Source: CAD feature listing. Evaluate the final solid. Frame: model axes, mm. A direction names the side the tool comes from. Coordinates: 2 decimals unless noted, no trailing zeros. Write each loop counter-clockwise with the first axis right and the second up, starting at its lowest first coordinate (ties: lowest second). Pieces come first, ordered by that corner, then holes. Notation, with made-up numbers: M -8.5,45 L -0.5,45 A20 cw -0.5,74 Z; hole C 47.5,0.25 d8. An arc over 180 degrees is marked long. Write item = value, one per line. Start each with the question number.
1. Section query C-C (z = 0). Output: boundary loops of the cut face in (x, y).
2. Access query for faces 3 (the face through (9.593, 4.93, 1.956)), 4 (the face through (1.26, 14.93, -0.17)). Directions: +Z, -Z, +X, -X, +Y, -Y. A direction counts if a zero-diameter tool reaches every point of the face in a straight line with its end or side. Return the directions, or none.
3. Section query D-D (z = 10). Output: boundary loops of the cut face in (x, y).
4. Line query: line 1 along X through (y, z) = (12.5, 0); line 2 along Y through (x, z) = (31, 13.5); line 3 along Z through (x, y) = (-1, 13.5). Output: solid intervals per line, ascending.
5. Section query A-A (x = 0). Output: boundary loops of the cut face in (y, z), then the cut area to 3 significant figures.
6. Pull-direction query (Z, two-part tool) for faces 1 (the face through (9.55, 4.93, -1.97)), 2 (the face through (18, 10, -18)); classes: pulls with the +Z half, pulls with the -Z half, needs draft (parallel to the pull), parting line crosses it, or undercut.
7. Pin query (flat end, axial travel): pin 1 Ø6 at (y, z) = (8, -5) entering from +X; pin 2 Ø2.5 at (y, z) = (6.5, 0) entering from +X; pin 3 Ø5 at (y, z) = (2.5, -17) entering from -X. Return the tip coordinate at first contact, or that it passes through.
```python
from build123d import *

# Parameters (mm, degrees)
SKETCH1_R           = 25
BOSS_EXTRUDE1_DEPTH = 10
SKETCH2_R           = 34
SKETCH2_R_2         = 1.27
BOSS_EXTRUDE2_DEPTH = 10
SKETCH3_R           = 3
CUT_EXTRUDE1_DEPTH  = 53.076866265


with BuildPart() as part:
    # Sketch1 → Boss-Extrude1 (new body)
    with BuildSketch(Plane(origin=(0, 0, 0), x_dir=(1, 0, 0), z_dir=(0, 1, 0))):
        with Locations(Location((0, 0, 0), (0, 0, 270))):
            Circle(SKETCH1_R)
        with BuildLine():
            Line((-1.5, 11), (1.5, 11))
            Line((1.5, 11), (2.425924848, 8.146464793))
            ThreePointArc((2.425924848, 8.146464793), (3.252809175, 7.852976026), (4.045032587, 7.475808409))
            Line((4.045032587, 7.475808409), (6.717514421, 8.838834765))
            Line((6.717514421, 8.838834765), (8.838834765, 6.717514421))
            Line((8.838834765, 6.717514421), (7.475808409, 4.045032587))
            ThreePointArc((7.475808409, 4.045032587), (7.852976026, 3.252809175), (8.146464793, 2.425924848))
            Line((8.146464793, 2.425924848), (11, 1.5))
            Line((11, 1.5), (11, -1.5))
            Line((11, -1.5), (8.146464793, -2.425924848))
            ThreePointArc((8.146464793, -2.425924848), (7.852976026, -3.252809175), (7.475808409, -4.045032587))
            Line((7.475808409, -4.045032587), (8.838834765, -6.717514421))
            Line((8.838834765, -6.717514421), (6.717514421, -8.838834765))
            Line((6.717514421, -8.838834765), (4.045032587, -7.475808409))
            ThreePointArc((4.045032587, -7.475808409), (3.252809175, -7.852976026), (2.425924848, -8.146464793))
            Line((2.425924848, -8.146464793), (1.5, -11))
            Line((1.5, -11), (-1.5, -11))
            Line((-1.5, -11), (-2.425924848, -8.146464793))
            ThreePointArc((-2.425924848, -8.146464793), (-3.252809175, -7.852976026), (-4.045032587, -7.475808409))
            Line((-4.045032587, -7.475808409), (-6.717514421, -8.838834765))
            Line((-6.717514421, -8.838834765), (-8.838834765, -6.717514421))
            Line((-8.838834765, -6.717514421), (-7.475808409, -4.045032587))
            ThreePointArc((-7.475808409, -4.045032587), (-7.852976026, -3.252809175), (-8.146464793, -2.425924848))
            Line((-8.146464793, -2.425924848), (-11, -1.5))
            Line((-11, -1.5), (-11, 1.5))
            Line((-11, 1.5), (-8.146464793, 2.425924848))
            ThreePointArc((-8.146464793, 2.425924848), (-7.852976026, 3.252809175), (-7.475808409, 4.045032587))
            Line((-7.475808409, 4.045032587), (-8.838834765, 6.717514421))
            Line((-8.838834765, 6.717514421), (-6.717514421, 8.838834765))
            Line((-6.717514421, 8.838834765), (-4.045032587, 7.475808409))
            ThreePointArc((-4.045032587, 7.475808409), (-3.252809175, 7.852976026), (-2.425924848, 8.146464793))
            Line((-2.425924848, 8.146464793), (-1.5, 11))
        make_face(mode=Mode.SUBTRACT)
    extrude(amount=BOSS_EXTRUDE1_DEPTH)

    # Sketch2 → Boss-Extrude2 (add)
    with BuildSketch(Plane(origin=(0, 10, 0), x_dir=(1, 0, 0), z_dir=(0, 1, 0))):
        with Locations(Location((0, 0, 0), (0, 0, 270))):
            Circle(SKETCH2_R)
        with Locations(Location((0, 0, 0), (0, 0, 270))):
            Circle(SKETCH2_R_2, mode=Mode.SUBTRACT)
    extrude(amount=BOSS_EXTRUDE2_DEPTH)

    # Sketch3 → Cut-Extrude1 (cut, through all)
    with BuildSketch(Plane(origin=(0, 20, 0), x_dir=(1, 0, 0), z_dir=(0, 1, 0))):
        with Locations(Location((-5, 0, 0), (0, 0, 270))):
            Circle(SKETCH3_R)
    extrude(amount=-CUT_EXTRUDE1_DEPTH, mode=Mode.SUBTRACT)


solid = part.part
```
Results are:
q1.outline = M -34,10 L -25,10 L -25,0 L -11,0 L -11,10 L -8,10 L -8,20 L -34,20 Z; M -2,10 L -1.27,10 L -1.27,20 L -2,20 Z; M 1.27,10 L 11,10 L 11,0 L 25,0 L 25,10 L 34,10 L 34,20 L 1.27,20 Z
q2.face_3 = -Y
q2.face_4 = +Y, -Y
q3.outline = M -32.5,10 L -22.91,10 L -22.91,0 L -1.82,0 L -1.82,10 L 1.82,10 L 1.82,0 L 22.91,0 L 22.91,10 L 32.5,10 L 32.5,20 L -32.5,20 Z
q4.line_1 = -34 to -8, -2 to -1.27, 1.27 to 34
q4.line_2 = 10 to 20
q4.line_3 = -33.99 to -0.78, 0.78 to 33.99
q5.outline = M 0,-25 L 10,-25 L 10,-34 L 20,-34 L 20,-1.27 L 10,-1.27 L 10,-11 L 0,-11 Z; M 0,11 L 10,11 L 10,1.27 L 20,1.27 L 20,34 L 10,34 L 10,25 L 0,25 Z
q5.area = 935 mm^2
q6.face_1 = undercut
q6.face_2 = needs draft
q7.pin_1 = 33.89
q7.pin_2 = 25
q7.pin_3 = -20.37
